The model under review builds one solid part; all positions refer to its coordinate system, in mm. A direction names the side the tool comes from. Coordinates: 2 decimals unless noted, no trailing zeros. Order: outer loops, then holes, each group sorted by start corner. A loop starts at its lowest first (then second) coordinate and runs counter-clockwise, first axis right, second up.
Autodesk Inventor part; units mm, degrees
ref_plane "YZ Plane" through (0, 0, 0) normal (1, 0, 0) x (0, 1, 0)
ref_plane "XZ Plane" through (0, 0, 0) normal (0, 1, 0) x (-1, 0, 0)
ref_plane "XY Plane" through (0, 0, 0) normal (0, 0, 1) x (1, 0, 0)
sketch "スケッチ1" plane through (0, 0, 0) normal (0, 0, 1) x (1, 0, 0)
  line L0 (0, 0) -> (10, 0)
  line L1 (10, 0) -> (10, -80)
  line L2 (10, -80) -> (0, -80)
  line L3 (0, -80) -> (0, 0)
  dimension "d0" = 10
  dimension "d1" = 80
extrude "押し出し1" add sketch "スケッチ1" along normal blind 1.5
fillet "フィレット1" radius 4 2 edges at (10, 0, 0.75) (0, 0, 0.75)
sketch "スケッチ9" plane through (0, -80, 0) normal (0, -1, 0) x (1, 0, 0)
  line L0 (0, 0) -> (20, 0)
  line L1 (20, 0) -> (20, 1.5)
  line L2 (20, 1.5) -> (0, 1.5)
  line L3 (0, 1.5) -> (0, 0)
  line L4 (10, 0) -> (10, 1.5)
  line L5 (10, 0) -> (0, 0)
  dimension "d35" = 20
  dimension "d36" = 1.5
  dimension "d37" = 10
  dimension "d38" = 0
extrude "押し出し8" add sketch "スケッチ9" along normal blind 10
sketch "スケッチ10" plane through (0, 0, 1.5) normal (0, 0, 1) x (1, 0, 0)
  line L0 (20, -90) -> (0, -90)
  line L1 (0, -4) -> (0, -90)
  point P0 (0, 0)
  point P1 (5, -85)
  point P2 (15, -85)
  dimension "d41" = 10
  dimension "d42" = 5
  dimension "d43" = 5
hole "穴2" at (5, -85, 1.5) at (15, -85, 1.5) direction (0, 0, -1) diameter 3.1 end through all
properties part number "Fork 1 left ver2c" material "アルミニウム 5052 H32"
(1) Insertion check: pin 1 Ø0.8 at (y, z) = (-58, 0.5) entering from +X; pin 2 Ø0.8 at (x, z) = (15, 1) entering from +Y. Each pin has a flat end and moves straight along its axis. Give the tip position at first contact, or say it passes through.
(2) Consider section D-D (y = -5). Give the boundary of the cut face in (x, z).
(3) The part is to be moulded in two halves that separate along Y. For faces 3 (the face through (15, -80, 1)), 4 (the face through (14.534, -86.478, 0.74)), 5 (the face through (10, -90, 1)), say which applies: +Y half, -Y half, draft (parallel to the pull), parting line (faces both ways), or undercut.
(4) Wall thickness on line 1 (X direction, y = -85, z = 0.85); line 2 (Y direction, x = 5, z = 0.65); line 3 (Y direction, x = 15, z = 0.6): over which ranges is each line inside the solid? List them lowest first.
(5) Consider section B-B (x = 5). Give the boundary of the cut face in (y, z).
(6) Tool access review of faces 1 (the face through (10, -41, 1)), 2 (the face through (5, 0, 1)): name each direction out of +Z, -Z, +X, -X, +Y, -Y from which nothing blocks a thin tool from reaching the whole face with its end or side.
(7) Consider section C-C (y = -85). Give the boundary of the cut face in (x, z).
(8) Consider section A-A (z = 0.9). Give the boundary of the cut face in (x, y), then the cut area to 3 significant figures.
Findings:
1. pin 1: stops at x = 10
1. pin 2: stops at y = -80
2. outline: (0, 0) - (10, 0) - (10, 1.5) - (0, 1.5) - close
3. face 3: +Y half
3. face 4: undercut
3. face 5: -Y half
4. line 1: x = 0 to 3.45, 6.55 to 13.45, 16.55 to 20
4. line 2: y = -90 to -86.55, -83.45 to 0
4. line 3: y = -90 to -86.55, -83.45 to -80
5. outline: (-90, 0) - (-86.55, 0) - (-86.55, 1.5) - (-90, 1.5) - close; (-83.45, 0) - (0, 0) - (0, 1.5) - (-83.45, 1.5) - close
6. face 1: +Z, -Z, +X, +Y
6. face 2: +Z, -Z, +X, -X, +Y
7. outline: (0, 0) - (3.45, 0) - (3.45, 1.5) - (0, 1.5) - close; (6.55, 0) - (13.45, 0) - (13.45, 1.5) - (6.55, 1.5) - close; (16.55, 0) - (20, 0) - (20, 1.5) - (16.55, 1.5) - close
8. outline: (0, -90) - (20, -90) - (20, -80) - (10, -80) - (10, -4) arc R4 ccw to (6, 0) - (4, 0) arc R4 ccw to (0, -4) - close; hole circle Ø3.1 at (5, -85); hole circle Ø3.1 at (15, -85)
8. area: 978 mm2
